Autodesk Fusion 360 part; units mm, degrees
sketch "Sketch1" plane through (0, 0, 0) normal (0, 0, 1) x (1, 0, 0)
sketch "Sketch2" plane through (0, 0, 0) normal (0, 0, 1) x (1, 0, 0)
  line L0 (6, 14) -> (-6, 14)
  line L1 (-6, 14) -> (-6, -14)
  line L2 (-6, -14) -> (6, -14)
  line L3 (6, -14) -> (6, 14)
  line L4 (6, 14) -> (-6, -14) construction
  line L5 (-6, 14) -> (6, -14) construction
  line L6 (-3, 3) -> (3, 3)
  line L7 (3, 3) -> (3, -3)
  line L8 (3, -3) -> (-3, -3)
  line L9 (-3, -3) -> (-3, 3)
  line L10 (-3, 3) -> (3, -3) construction
  line L11 (3, 3) -> (-3, -3) construction
  line L12 (5, -5) -> (-5, -5)
  line L13 (-5, -5) -> (-5, 5)
  line L14 (-5, 5) -> (5, 5)
  line L15 (5, 5) -> (5, -5)
  dimension "d10" = 12
  dimension "d11" = 28
  dimension "d12" = 6
  dimension "d13" = 6
  dimension "d14" = -2
extrude "Extrude3" add sketch "Sketch2" along normal blind 2 contours L0 L1 L2 L3 | L6 L7 L8 L9 | L12 L13 L14 L15
extrude "Extrude4" add sketch "Sketch2" along normal blind 13 contours L6 L7 L8 L9 | L12 L13 L14 L15
extrude "Extrude5" cut sketch "Sketch2" along normal blind 9.5 contours L6 L7 L8 L9
sketch "Sketch3" plane through (0, -5, 0) normal (0, -1, 0) x (1, 0, 0)
  line L0 (-5, 2) -> (5, 2)
  line L1 (5, 2) -> (5, 13)
  line L2 (5, 13) -> (-5, 13)
  line L3 (-5, 13) -> (-5, 2)
  line L4 (0, 13) -> (0, 11.5)
  line L5 (0, 11.5) -> (0, 5)
  line L6 (0, 5) -> (0, 2)
  line L7 (0, 11.5) -> (0, 8.25)
  circle A0 centre (0, 8.25) radius 3.25
  circle A1 centre (0, 8.25) radius 4.75
  line L8 (0, 8.25) -> (5, 8.25)
  line L9 (5, 8.25) -> (-5, 8.25)
  dimension "d21" = 1.5
  dimension "d22" = 6.5
  dimension "d23" = 3.25
  dimension "d24" = 6.5
  dimension "d25" = 1.5
extrude "Extrude6" cut sketch "Sketch3" against normal blind 12 contours L5 A0 L9 | L5 A0 L8 L9 | L5 L7 A0 L9 | L5 L7 A0 L8 L9
extrude "Extrude7" cut sketch "Sketch3" against normal blind 10 contours L2 L3 A1 L9 | L1 L2 A1 L8 L9
sketch "Sketch4" plane through (0, 5, 0) normal (0, 1, 0) x (-1, 0, 0)
  line L0 (-4.75, 8.25) -> (-5, 8.25)
  line L1 (-5, 8.25) -> (-5, 2)
  line L2 (-5, 2) -> (5, 2)
  line L3 (5, 2) -> (5, 8.25)
  line L4 (5, 8.25) -> (4.75, 8.25)
  arc A0 (4.75, 8.25) -> (-4.75, 8.25) centre (0, 8.25) ccw
  circle A1 centre (0, 8.25) radius 3.25
  line L5 (4.75, 8.25) -> (5, 2)
  line L6 (-5, 2) -> (-4.75, 8.25)
extrude "Extrude8" cut sketch "Sketch4" against normal blind 10 contours L0 L1 L6 | L3 L4 L5
sketch "Sketch5" plane through (0, 0, 0) normal (0, 0, 1) x (1, 0, 0)
  line L0 (3, 3) -> (-3, 3)
  line L1 (-3, 3) -> (-3, -3)
  line L2 (-3, -3) -> (3, -3)
  line L3 (3, -3) -> (3, 3)
  line L4 (3, 3) -> (-3, -3) construction
  line L5 (-3, 3) -> (3, -3) construction
  dimension "d32" = 6
  dimension "d33" = 6
ref_plane "WorkPlane1" through (0, 0, 13) normal (0, 0, 1) x (1, 0, 0)
sketch "Sketch6" plane through (0, 0, 13) normal (0, 0, 1) x (1, 0, 0)
  line L0 (5, 3) -> (-5, 3)
  line L1 (-5, 3) -> (-5, -3)
  line L2 (-5, -3) -> (5, -3)
  line L3 (5, -3) -> (5, 3)
  line L4 (5, 3) -> (-5, -3) construction
  line L5 (-5, 3) -> (5, -3) construction
  dimension "d35" = 10
  dimension "d36" = 6
sketch "Sketch7" plane through (0, 0, 13) normal (0, 0, 1) x (1, 0, 0)
  line L0 (-5, 5) -> (5, 5)
  line L1 (5, 5) -> (5, -5)
  line L2 (5, -5) -> (-5, -5)
  line L3 (-5, -5) -> (-5, 5)
  line L4 (-5, 5) -> (5, -5) construction
  line L5 (5, 5) -> (-5, -5) construction
  line L6 (5, -5) -> (-5, -5)
  line L7 (-5, -5) -> (-5, -3)
  line L8 (-5, -3) -> (5, -3)
  line L9 (5, -3) -> (5, -5)
  line L10 (5, 5) -> (5, 5)
  line L11 (5, 5) -> (5, 3)
  line L12 (5, 3) -> (5, 3)
  line L13 (5, 3) -> (5, 5)
  line L14 (-5, 3.0009) -> (5, 3.0009)
  line L15 (5, 3.0009) -> (5, 5)
  line L16 (5, 5) -> (-5, 5)
  line L17 (-5, 5) -> (-5, 3.0009)
  dimension "d37" = 10
extrude "Extrude9" cut sketch "Sketch7" against normal blind 5 contours L0 L1 L3 L11 L13 L14 L15 L16 L17 | L1 L2 L3 L6 L7 L8 L9
Geometry check sheet. Reference: the model listing, model coordinates, mm. A direction names the side the tool comes from. Coordinates: 2 decimals unless noted, no trailing zeros. Order: outer loops, then holes, each group sorted by start corner. A loop starts at its lowest first (then second) coordinate and runs counter-clockwise, first axis right, second up. Notation, with made-up numbers: M 67.5,26.25 L 117.5,26.25 A22 ccw 117.5,58.25 Z; hole C 61.5,-38 d4. An arc over 180 degrees is marked long. One line per question, with ' | ' between items. Start each with the question number.
Item 1: Cross-section at A-A on x = 1.5. Enter the section's corners in (y, z), then the cut area to 3 significant figures.
Item 2: Material ranges on L1, parallel to X at y = 2.75, z = 8.25; L2, parallel to Y at x = 1.5, z = 4; L3, parallel to Y at x = -4.75, z = 4.5, recorded low to high. Write a range as [from, to].
Item 3: Cross-section at D-D on x = 0. Enter the section's corners in (y, z).
Item 4: Draft check along Y on faces 1 (the flat face through (0, 14, 1)), 2 (the flat face through (-4, -4, 8)), 3 (the flat face through (0, -3, 3)). Enter one of: pulls with the +Y half, pulls with the -Y half, needs draft (parallel to the pull), parting line crosses it, or undercut.
Item 5: Gauge pin test, flat ends, axial feed: pin 1 (1.2 mm diameter, centred on x = -4, y = -4, fed in from +Z); pin 2 (4 mm diameter, centred on x = 3, z = 6.5, fed in from +Y); pin 3 (5.5 mm diameter, centred on x = 1.5, z = 10.5, fed in from -Y). Record the tip position at first contact, or that the pin passes through.
Item 6: Cross-section at B-B on z = 3.5. Enter the section's corners in (x, y), then the cut area to 3 significant figures.
Item 7: Set-up check for faces 4 (the flat face through (0, 3, 3)), 5 (the flat face through (4.877, 0.07, 5.081)), 6 (the flat face through (4, -4, 8)), 7 (the flat face through (-4, 4, 8)): record each of +Z, -Z, +X, -X, +Y, -Y from which the full face is reachable in a straight line by a thin tool's end or side.
Item 8: Cross-section at C-C on y = 1. Enter the section's corners in (x, z), then the cut area to 3 significant figures.
Findings:
1) outline: M -14,0 L -3,0 L -3,5.37 L -5,5.37 L -5,2 L -14,2 Z; M -3,11.13 L 3,11.13 L 3,12.76 L -3,12.76 Z; M 3,0 L 14,0 L 14,2 L 5,2 L 5,5.37 L 3,5.37 Z | area: 67.2 mm²
2) L1: x = [-4.75, -3.25], [3.25, 4.75] | L2: y = [-5, -3], [3, 5] | L3: y = [-5, 5]
3) outline: M -14,0 L -3,0 L -3,5 L -5,5 L -5,2 L -14,2 Z; M -3,11.5 L 3,11.5 L 3,13 L -3,13 Z; M 3,0 L 14,0 L 14,2 L 5,2 L 5,5 L 3,5 Z
4) face 1: pulls with the +Y half | face 2: needs draft | face 3: undercut
5) pin 1: stops at z = 8 | pin 2: stops at y = 5 | pin 3: stops at y = -3
6) outline: M -4.94,-5 L 4.94,-5 L 4.94,5 L -4.94,5 Z; hole M -3,-3 L 3,-3 L 3,3 L -3,3 Z | area: 62.8 mm²
7) face 4: -Z | face 5: +Z, +X, +Y, -Y | face 6: +Z, +X, -X, -Y | face 7: +Z, +X, -X, +Y
8) outline: M -6,0 L -3,0 L -3,7 A3.25 cw long 3,7 L 3,0 L 6,0 L 6,2 L 5,2 L 4.75,8.25 A4.75 ccw -4.75,8.25 L -5,2 L -6,2 Z | area: 53.9 mm²
